Verification items for the finished model (mm, model axes). Give positions to 0.01 mm unless a question says otherwise; leave off trailing zeros. Write each loop counter-clockwise with the first axis right and the second up, starting at its lowest first coordinate (ties: lowest second). Pieces come first, ordered by that corner, then holes.
from build123d import *

# Parameters (mm, degrees)
F0_W     = 24
F0_H     = 1.6
F1_DEPTH = 1.6
F2_SIZE2 = 1
F2_SIZE  = 1
F3_SIZE  = 1


with BuildPart() as f1:
    # F0 (on Top) → F1 (new body)
    with BuildSketch(Plane.XY):
        with Locations((-17.850905, 7.283434)):
            Rectangle(F0_W, F0_H)
    extrude(amount=F1_DEPTH)

    # F2
    f2_edges = [f1.edges().sort_by_distance(p)[0] for p in [
        (-29.850905, 8.083434, 0.8),
    ]]
    chamfer(f2_edges, length=F2_SIZE, length2=F2_SIZE2)

    # F3
    f3_edges = [f1.edges().sort_by_distance(p)[0] for p in [
        (-5.850905, 8.083434, 0.8),
    ]]
    chamfer(f3_edges, length=F3_SIZE)


solid = f1.part
Item 1: Sectioned sample at B-B on y = 7.4. Record the cut outline in (x, z), then the cut area to 3 significant figures.
Answer key:
outline: (-29.53, 0) - (-6.17, 0) - (-6.17, 1.6) - (-29.53, 1.6) - close
area: 37.4 mm2
Item 2: Sectioned sample at A-A on z = 0.6. Record the cut outline in (x, y), then the cut area to 3 significant figures.
Answer key:
outline: (-29.85, 6.48) - (-5.85, 6.48) - (-5.85, 7.08) - (-6.85, 8.08) - (-28.85, 8.08) - (-29.85, 7.08) - close
area: 37.4 mm2
Item 3: Scan lines: line 1 along X through (y, z) = (7.4, 1.05); line 2 along X through (y, z) = (8.05, 1.2). Record each from-to range of solid material in increasing order.
Answer key:
line 1: x = -29.53 to -6.17
line 2: x = -28.88 to -6.82
